```python
from build123d import *

# Parameters (mm, degrees)
SKETCH_W        = 18
SKETCH_H        = 23.5
SKETCH_R        = 0.5
PAD_DEPTH       = 1.6
SKETCH001_R     = 0.5
POCKET_DEPTH    = 5
SKETCH002_W     = 8.98
SKETCH002_H     = 7.5
PAD001_DEPTH    = 3.28
SKETCH003_W     = 9.38
SKETCH003_H     = 4.38
POCKET001_DEPTH = 7
SKETCH004_W     = 6.69
SKETCH004_H     = 1.2
POCKET002_DEPTH = 6
SKETCH005_W     = 3.4
SKETCH005_H     = 4.3
PAD002_DEPTH    = 1.5
SKETCH006_W     = 1.9
SKETCH006_H     = 1.8
PAD003_DEPTH    = 1
PAD004_DEPTH    = 0.5


with BuildPart() as part:
    # Sketch → Pad (new body)
    with BuildSketch(Plane.XY):
        with Locations((9, 11.75)):
            Rectangle(SKETCH_W, SKETCH_H)
        with Locations((1.38, 21.91)):
            Circle(SKETCH_R, mode=Mode.SUBTRACT)
        with Locations((1.38, 19.37)):
            Circle(SKETCH_R, mode=Mode.SUBTRACT)
        with Locations((1.38, 16.83)):
            Circle(SKETCH_R, mode=Mode.SUBTRACT)
        with Locations((1.38, 14.29)):
            Circle(SKETCH_R, mode=Mode.SUBTRACT)
        with Locations((1.38, 11.75)):
            Circle(SKETCH_R, mode=Mode.SUBTRACT)
        with Locations((1.38, 9.21)):
            Circle(SKETCH_R, mode=Mode.SUBTRACT)
        with Locations((1.38, 6.67)):
            Circle(SKETCH_R, mode=Mode.SUBTRACT)
        with Locations((1.38, 4.13)):
            Circle(SKETCH_R, mode=Mode.SUBTRACT)
        with Locations((1.38, 1.59)):
            Circle(SKETCH_R, mode=Mode.SUBTRACT)
        with Locations((16.62, 21.91)):
            Circle(SKETCH_R, mode=Mode.SUBTRACT)
        with Locations((16.62, 19.37)):
            Circle(SKETCH_R, mode=Mode.SUBTRACT)
        with Locations((16.62, 16.83)):
            Circle(SKETCH_R, mode=Mode.SUBTRACT)
        with Locations((16.62, 14.29)):
            Circle(SKETCH_R, mode=Mode.SUBTRACT)
        with Locations((16.62, 11.75)):
            Circle(SKETCH_R, mode=Mode.SUBTRACT)
        with Locations((16.62, 9.21)):
            Circle(SKETCH_R, mode=Mode.SUBTRACT)
        with Locations((16.62, 6.67)):
            Circle(SKETCH_R, mode=Mode.SUBTRACT)
        with Locations((16.62, 4.13)):
            Circle(SKETCH_R, mode=Mode.SUBTRACT)
        with Locations((16.62, 1.59)):
            Circle(SKETCH_R, mode=Mode.SUBTRACT)
        with Locations((14.08, 1.59)):
            Circle(SKETCH_R, mode=Mode.SUBTRACT)
        with Locations((11.54, 1.59)):
            Circle(SKETCH_R, mode=Mode.SUBTRACT)
        with Locations((9, 1.59)):
            Circle(SKETCH_R, mode=Mode.SUBTRACT)
        with Locations((6.46, 1.59)):
            Circle(SKETCH_R, mode=Mode.SUBTRACT)
        with Locations((3.92, 1.59)):
            Circle(SKETCH_R, mode=Mode.SUBTRACT)
    extrude(amount=PAD_DEPTH)

    # Sketch001 (on Face29 of Pad) → Pocket (cut)
    with BuildSketch(Plane.XY.offset(1.6)):
        with Locations((0, 21.91)):
            Circle(SKETCH001_R)
        with Locations((0, 19.37)):
            Circle(SKETCH001_R)
        with Locations((0, 16.83)):
            Circle(SKETCH001_R)
        with Locations((0, 14.29)):
            Circle(SKETCH001_R)
        with Locations((0, 11.75)):
            Circle(SKETCH001_R)
        with Locations((0, 9.21)):
            Circle(SKETCH001_R)
        with Locations((0, 6.67)):
            Circle(SKETCH001_R)
        with Locations((0, 4.13)):
            Circle(SKETCH001_R)
        with Locations((0, 1.59)):
            Circle(SKETCH001_R)
        with Locations((18, 21.91)):
            Circle(SKETCH001_R)
        with Locations((18, 19.37)):
            Circle(SKETCH001_R)
        with Locations((18, 16.83)):
            Circle(SKETCH001_R)
        with Locations((18, 14.29)):
            Circle(SKETCH001_R)
        with Locations((18, 11.75)):
            Circle(SKETCH001_R)
        with Locations((18, 9.21)):
            Circle(SKETCH001_R)
        with Locations((18, 6.67)):
            Circle(SKETCH001_R)
        with Locations((18, 4.13)):
            Circle(SKETCH001_R)
        with Locations((18, 1.59)):
            Circle(SKETCH001_R)
        with Locations((3.92, 0.21)):
            Circle(SKETCH001_R)
        with Locations((6.46, 0.21)):
            Circle(SKETCH001_R)
        with Locations((9, 0.21)):
            Circle(SKETCH001_R)
        with Locations((11.54, 0.21)):
            Circle(SKETCH001_R)
        with Locations((14.08, 0.21)):
            Circle(SKETCH001_R)
    extrude(amount=-POCKET_DEPTH, mode=Mode.SUBTRACT)

    # Sketch002 (on Face3 of Pocket) → Pad001 (join)
    with BuildSketch(Plane.XY.offset(1.6)):
        with Locations((9, 20.41)):
            Rectangle(SKETCH002_W, SKETCH002_H)
    extrude(amount=PAD001_DEPTH)

    # Sketch003 (on Face80 of Pad001) → Pocket001 (cut)
    with BuildSketch(Plane(origin=(0, 24.16, 0), x_dir=(-1, 0, 0), z_dir=(0, 1, 0))):
        with Locations((-9, 3.69)):
            Rectangle(SKETCH003_W, SKETCH003_H)
        with BuildLine():
            Line((-11.91, 1.6), (-6.09, 1.6))
            ThreePointArc((-6.09, 1.6), (-4.972771, 2.062771), (-4.51, 3.18))
            Line((-4.51, 3.18), (-4.51, 3.3))
            ThreePointArc((-4.51, 3.3), (-4.972771, 4.417229), (-6.09, 4.88))
            Line((-6.09, 4.88), (-11.91, 4.88))
            ThreePointArc((-11.91, 4.88), (-13.027229, 4.417229), (-13.49, 3.3))
            Line((-13.49, 3.3), (-13.49, 3.18))
            ThreePointArc((-13.49, 3.18), (-13.027229, 2.062771), (-11.91, 1.6))
        make_face(mode=Mode.SUBTRACT)
    extrude(amount=-POCKET001_DEPTH, mode=Mode.SUBTRACT)

    # Sketch004 (on Face83 of Pocket001) → Pocket002 (cut)
    with BuildSketch(Plane(origin=(0, 24.16, 0), x_dir=(-1, 0, 0), z_dir=(0, 1, 0))):
        with BuildLine():
            Line((-12.04, 1.85), (-5.96, 1.85))
            ThreePointArc((-5.96, 1.85), (-5.111472, 2.201472), (-4.76, 3.05))
            Line((-4.76, 3.05), (-4.76, 3.43))
            ThreePointArc((-4.76, 3.43), (-5.111472, 4.278528), (-5.96, 4.63))
            Line((-5.96, 4.63), (-12.04, 4.63))
            ThreePointArc((-12.04, 4.63), (-12.888528, 4.278528), (-13.24, 3.43))
            Line((-13.24, 3.43), (-13.24, 3.05))
            ThreePointArc((-13.24, 3.05), (-12.888528, 2.201472), (-12.04, 1.85))
        make_face()
        with Locations((-9, 3.24)):
            Rectangle(SKETCH004_W, SKETCH004_H, mode=Mode.SUBTRACT)
    extrude(amount=-POCKET002_DEPTH, mode=Mode.SUBTRACT)

    # Sketch005 (on Face4 of Pocket002) → Pad002 (join)
    with BuildSketch(Plane.XY.offset(1.6)):
        with Locations((4.6, 7.55)):
            Rectangle(SKETCH005_W, SKETCH005_H)
        with Locations((13.7, 7.55)):
            Rectangle(SKETCH005_W, SKETCH005_H)
    extrude(amount=PAD002_DEPTH)

    # Sketch006 (on Face4 of Pad002) → Pad003 (join)
    with BuildSketch(Plane.XY.offset(1.6)):
        with Locations((9.15, 8.1)):
            Rectangle(SKETCH006_W, SKETCH006_H)
    extrude(amount=PAD003_DEPTH)

    # Sketch007 (on Face106 of Pad003) → Pad004 (join)
    with BuildSketch(Plane.XY.offset(3.1)):
        with BuildLine():
            ThreePointArc((12.7, 7.05), (13.7, 6.05), (14.7, 7.05))
            Line((14.7, 7.05), (14.7, 8.05))
            ThreePointArc((14.7, 8.05), (13.7, 9.05), (12.7, 8.05))
            Line((12.7, 7.05), (12.7, 8.05))
        make_face()
        with BuildLine():
            ThreePointArc((3.6, 7.05), (4.6, 6.05), (5.6, 7.05))
            Line((5.6, 7.05), (5.6, 8.05))
            ThreePointArc((5.6, 8.05), (4.6, 9.05), (3.6, 8.05))
            Line((3.6, 7.05), (3.6, 8.05))
        make_face()
    extrude(amount=PAD004_DEPTH)


solid = part.part
```
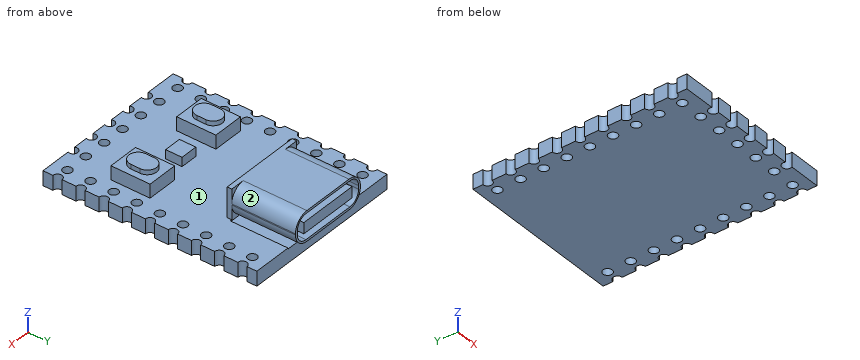
Could you check a few things on this model? Use its own coordinates, in mm. Face numbers are marked on the shaded views. Coordinates: 2 decimals unless noted, no trailing zeros. Write each loop counter-clockwise with the first axis right and the second up, starting at its lowest first coordinate (ties: lowest second). Pieces come first, ordered by that corner, then holes. Notation, with made-up numbers: (16, -3.5) -> (36, -3.5) arc R30 ccw to (36, 18.5) -> close; hole circle Ø7 at (-27, 8.25). An arc over 180 degrees is marked (long way). One line per question, with ' | ' between items. Start each with the question number.
1. Please list where these lines run through material, in increasing order: line 1 along X through (y, z) = (0.21, 0.65); line 2 along X through (y, z) = (6.5, 0.9); line 3 along Z through (x, y) = (1, 5.25).
2. Thinking about a two-plate mould opening in Y: for the marked faces 1 and 2, which applies, pulls with the +Y half, pulls with the -Y half, needs draft (parallel to the pull), parting line crosses it, or undercut?
3. If we section it at D-D (y = 10): Please give me the cut outline in (x, z).
4. If we section it at A-A (y = 21): Please give me the cut outline in (x, z) (3 decimals), and give its area (3 significant figures).
5. If we section it at B-B (y = 4.13): Please give me the cut outline in (x, z), and give its area (3 significant figures).
6. Will these pins go through, and if not, where does the flat tip stop? P1, Ø0.5, axis at y = 8, z = 2, coming from the +X side; P2, Ø1.5, axis at x = 7.5, y = 14.5, coming from the +Z side; P3, Ø2.5, axis at y = 20.5, z = 3.5, coming from the +X side.
7. If we section it at C-C (z = 0.9): Count the separate pieces of the cut face and the enclosed holes in it, and give its area (3 significant figures).
Return value:
1) line 1: x = 0 to 3.42, 4.42 to 5.96, 6.96 to 8.5, 9.5 to 11.04, 12.04 to 13.58, 14.58 to 18 | line 2: x = 0.47 to 0.91, 1.85 to 16.15, 17.09 to 17.53 | line 3: z = 0 to 1.6
2) face 1: undercut | face 2: needs draft
3) outline: (0, 0) -> (18, 0) -> (18, 1.6) -> (0, 1.6) -> close
4) outline: (0, 0) -> (18, 0) -> (18, 1.6) -> (13.69, 1.6) -> (13.69, 1.5) -> (4.31, 1.5) -> (4.31, 1.6) -> (0, 1.6) -> close; (4.51, 3.18) arc R1.58 ccw to (6.09, 1.6) -> (11.91, 1.6) arc R1.58 ccw to (13.49, 3.18) -> (13.49, 3.3) arc R1.58 ccw to (11.91, 4.88) -> (6.09, 4.88) arc R1.58 ccw to (4.51, 3.3) -> close; (5.655, 2.64) -> (12.345, 2.64) -> (12.345, 3.84) -> (5.655, 3.84) -> close; hole (4.76, 3.05) arc R1.2 ccw to (5.96, 1.85) -> (12.04, 1.85) arc R1.2 ccw to (13.24, 3.05) -> (13.24, 3.43) arc R1.2 ccw to (12.04, 4.63) -> (5.96, 4.63) arc R1.2 ccw to (4.76, 3.43) -> close | area: 40.9 mm²
5) outline: (0.5, 0) -> (0.88, 0) -> (0.88, 1.6) -> (0.5, 1.6) -> close; (1.88, 0) -> (16.12, 0) -> (16.12, 1.6) -> (1.88, 1.6) -> close; (17.12, 0) -> (17.5, 0) -> (17.5, 1.6) -> (17.12, 1.6) -> close | area: 24.0 mm²
6) P1: stops at x = 15.4 | P2: stops at z = 1.6 | P3: stops at x = 13.49
7) separate pieces: 1 | enclosed holes: 23 | area: 395 mm²
